```python
from build123d import *

# Parameters (mm, degrees)
SKETCH_1_R      = 39.5
SKETCH_1_R_2    = 2.05
SKETCH_1_R_3    = 5.05
SKETCH_1_W      = 8.1
SKETCH_1_H      = 2.1
EXTRUDE_1_DEPTH = 2


with BuildPart() as part:
    # 草图1 → 凸台-拉伸1 (new body)
    with BuildSketch(Plane.XY):
        with Locations((0, 35.4)):
            Circle(SKETCH_1_R)
        Circle(SKETCH_1_R_2, mode=Mode.SUBTRACT)
        with Locations((0, 20)):
            Circle(SKETCH_1_R_2, mode=Mode.SUBTRACT)
        with Locations((0, 35.4)):
            Circle(SKETCH_1_R_3, mode=Mode.SUBTRACT)
        with Locations((-15, 20)):
            Rectangle(SKETCH_1_W, SKETCH_1_H, mode=Mode.SUBTRACT)
        with Locations((15, 20)):
            Rectangle(SKETCH_1_W, SKETCH_1_H, mode=Mode.SUBTRACT)
    extrude(amount=EXTRUDE_1_DEPTH)


solid = part.part
```
Source: CAD feature listing. Evaluate the final solid. Frame: model axes, mm. A direction names the side the tool comes from. Coordinates: 2 decimals unless noted, no trailing zeros. Order: outer loops, then holes, each group sorted by start corner. A loop starts at its lowest first (then second) coordinate and runs counter-clockwise, first axis right, second up. Notation, with made-up numbers: (-3, -36) - (19, -36) arc R19 cw to (19, -17) - close; hole circle Ø4 at (32, 71.5). An arc over 180 degrees is marked (long way). One line per item, written item: value.
1) Cut plane A-A on x = 0. Output: boundary loops of the cut face in (y, z), plus the area to 3 significant figures.
Computed values:
outline: (-4.1, 0) - (-2.05, 0) - (-2.05, 2) - (-4.1, 2) - close; (2.05, 0) - (17.95, 0) - (17.95, 2) - (2.05, 2) - close; (22.05, 0) - (30.35, 0) - (30.35, 2) - (22.05, 2) - close; (40.45, 0) - (74.9, 0) - (74.9, 2) - (40.45, 2) - close
area: 121 mm^2
2) Cut plane D-D on y = 20. Output: boundary loops of the cut face in (x, z), plus the area to 3 significant figures.
Computed values:
outline: (-36.37, 0) - (-19.05, 0) - (-19.05, 2) - (-36.37, 2) - close; (-10.95, 0) - (-2.05, 0) - (-2.05, 2) - (-10.95, 2) - close; (2.05, 0) - (10.95, 0) - (10.95, 2) - (2.05, 2) - close; (19.05, 0) - (36.37, 0) - (36.37, 2) - (19.05, 2) - close
area: 105 mm^2
3) Cut plane C-C on y = 35.4. Output: boundary loops of the cut face in (x, z), plus the area to 3 significant figures.
Computed values:
outline: (-39.5, 0) - (-5.05, 0) - (-5.05, 2) - (-39.5, 2) - close; (5.05, 0) - (39.5, 0) - (39.5, 2) - (5.05, 2) - close
area: 138 mm^2
4) Reachability of faces 4 (the face through (8, 36, 0)), 5 (the face through (-19.05, 20, 1)) from +Z, -Z, +X, -X, +Y, -Y: full face, straight path, thin tool, end or side. Return the list, or none.
Computed values:
face 4: -Z, +X, -X, +Y, -Y
face 5: +Z, -Z
5) Cut plane B-B on z = 1.7. Output: boundary loops of the cut face in (x, y).
Computed values:
outline: circle Ø79 at (0, 35.4); hole (-19.05, 18.95) - (-10.95, 18.95) - (-10.95, 21.05) - (-19.05, 21.05) - close; hole circle Ø10.1 at (0, 35.4); hole circle Ø4.1 at (0, 0); hole circle Ø4.1 at (0, 20); hole (10.95, 18.95) - (19.05, 18.95) - (19.05, 21.05) - (10.95, 21.05) - close
6) Ray query, line 1 (Y direction, x = 0, z = 1.5); line 2 (Y direction, x = 2.5, z = 0.1); line 3 (X direction, y = 19, z = 1.7). Return the intervals inside material, ascending. Write a range as [from, to].
Computed values:
line 1: y = [-4.1, -2.05], [2.05, 17.95], [22.05, 30.35], [40.45, 74.9]
line 2: y = [-4.02, 31.01], [39.79, 74.82]
line 3: x = [-35.93, -19.05], [-10.95, -1.79], [1.79, 10.95], [19.05, 35.93]
7) Contact query for flat-ended pins moving along their axis: pin 1 (1 mm diameter, centred on x = 14, z = 1, fed in from -Y); pin 2 (1 mm diameter, centred on x = 7, z = 0.5, fed in from +Y); pin 3 (1 mm diameter, centred on y = 20.5, z = 1, fed in from -X); pin 4 (3.5 mm diameter, centred on x = 0, y = 0, fed in from +Z). Output: stop coordinate, or through.
Computed values:
pin 1: stops at y = -1.72
pin 2: stops at y = 74.36
pin 3: stops at x = -36.78
pin 4: passes through
8) Mould query, pull axis Y, two halves, no side actions, for faces 1 (the face through (-0.7, 40.4, 1)), 2 (the face through (-29.11, 62.1, 0.99)), 3 (the face through (8, 36, 2)). Classes: released by +Y, released by -Y, zero draft, split by the parting line, or undercut.
Computed values:
face 1: undercut
face 2: split by the parting line
face 3: zero draft
